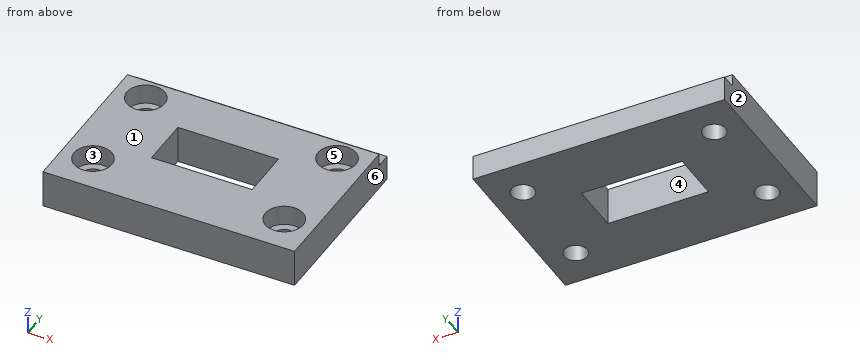
from build123d import *

# Parameters (mm, degrees)
SKETCH_1_W          = 100
SKETCH_1_H          = 70
EXTRUDE_1_DEPTH     = 15
SKETCH_2_W          = 100
SKETCH_2_H          = 6
CUT_EXTRUDE_1_DEPTH = 5
SKETCH_3_W          = 40
SKETCH_3_H          = 20
CUT_EXTRUDE_2_DEPTH = 63.84902545
SKETCH_4_R          = 7.5
CUT_EXTRUDE_3_DEPTH = 8
SKETCH_5_R          = 4.5
CUT_EXTRUDE_4_DEPTH = 63.84902545


with BuildPart() as part:
    # 草图1 → 凸台-拉伸1 (new body)
    with BuildSketch(Plane.XY):
        Rectangle(SKETCH_1_W, SKETCH_1_H)
    extrude(amount=EXTRUDE_1_DEPTH)

    # 草图2 → 切除-拉伸1 (cut)
    with BuildSketch(Plane.XY.offset(15)):
        with Locations((0, 32)):
            Rectangle(SKETCH_2_W, SKETCH_2_H)
    extrude(amount=-CUT_EXTRUDE_1_DEPTH, mode=Mode.SUBTRACT)

    # 草图3 → 切除-拉伸2 (cut, through all)
    with BuildSketch(Plane.XY):
        Rectangle(SKETCH_3_W, SKETCH_3_H)
    extrude(amount=CUT_EXTRUDE_2_DEPTH, mode=Mode.SUBTRACT)

    # 草图4 → 切除-拉伸3 (cut)
    with BuildSketch(Plane.XY.offset(15)):
        with Locations((38, 20)):
            Circle(SKETCH_4_R)
        with Locations((-38, 20)):
            Circle(SKETCH_4_R)
        with Locations((38, -20)):
            Circle(SKETCH_4_R)
        with Locations((-38, -20)):
            Circle(SKETCH_4_R)
    extrude(amount=-CUT_EXTRUDE_3_DEPTH, mode=Mode.SUBTRACT)

    # 草图5 → 切除-拉伸4 (cut, through all)
    with BuildSketch(Plane.XY.offset(15)):
        with Locations((38, 20)):
            Circle(SKETCH_5_R)
        with Locations((-38, 20)):
            Circle(SKETCH_5_R)
        with Locations((38, -20)):
            Circle(SKETCH_5_R)
        with Locations((-38, -20)):
            Circle(SKETCH_5_R)
    extrude(amount=-CUT_EXTRUDE_4_DEPTH, mode=Mode.SUBTRACT)


solid = part.part
The listing builds one solid part. Answer for the finished solid, in the listing's coordinates (mm). Face numbers are marked on the shaded views. A direction names the side the tool comes from. Coordinates: 2 decimals unless noted, no trailing zeros. Loops run counter-clockwise (first coordinate to the right, second up) from the corner with the lowest first, then second, coordinate; pieces in that order, holes last. Notation, with made-up numbers: (56, 44) -> (75, 44) arc R11 cw to (75, 53) -> close; hole circle Ø10 at (27.25, 20). An arc over 180 degrees is marked (long way). Answer in a Markdown table with one row per item. Add a question column.
1. For the marked faces 4, 5 and 6, determine the directions among +Z, -Z, +X, -X, +Y, -Y from which every point of the face is accessible in a straight line to the end or side of a thin tool.
2. The part is cut by section A-A, the plane x = -14. Write down the section's boundary in (y, z), then the cut area to 3 significant figures.
3. The part is cut by section B-B, the plane z = 8. Write down the section's boundary in (x, y).
4. Consider line 1 (Y direction, x = -38.5, z = 10.25); line 2 (Y direction, x = 38, z = 4); line 3 (Y direction, x = -13.5, z = 4). Determine where each line is inside the solid, lowest interval first. Write a range as [from, to].
5. The part is cut by section C-C, the plane y = -3. Write down the section's boundary in (x, z).
6. The part is cut by section D-D, the plane y = -18. Write down the section's boundary in (x, z).
7. Determine the mould class of the marked faces 1, 2 and 3 for opening direction X: +X half, -X half, draft (parallel to the pull), parting line (faces both ways), or undercut.
8. Flat-ended cylindrical pins translate along their axes: P1, Ø10.5, axis at x = -38, y = -20, coming from the +Z side; P2, Ø5, axis at x = -14.5, y = 33, coming from the +Z side; P3, Ø2.5, axis at x = 8.5, z = 13, coming from the +Y side. Find the tip coordinate at first contact, or state that the pin passes through.
Answer below:
| question | item | result |
|---|---|---|
| 1 | face 4 | +Z, -Z |
| 1 | face 5 | +Z |
| 1 | face 6 | +Z, -Z, +X, +Y, -Y |
| 2 | outline | (-35, 0) -> (-10, 0) -> (-10, 15) -> (-35, 15) -> close; (10, 0) -> (35, 0) -> (35, 10) -> (29, 10) -> (29, 15) -> (10, 15) -> close |
| 2 | area | 720 mm2 |
| 3 | outline | (-50, -35) -> (50, -35) -> (50, 35) -> (-50, 35) -> close; hole circle Ø15 at (-38, -20); hole circle Ø15 at (-38, 20); hole (-20, -10) -> (20, -10) -> (20, 10) -> (-20, 10) -> close; hole circle Ø15 at (38, -20); hole circle Ø15 at (38, 20) |
| 4 | line 1 | [-35, -27.48], [-12.52, 12.52], [27.48, 29] |
| 4 | line 2 | [-35, -24.5], [-15.5, 15.5], [24.5, 35] |
| 4 | line 3 | [-35, -10], [10, 35] |
| 5 | outline | (-50, 0) -> (-20, 0) -> (-20, 15) -> (-50, 15) -> close; (20, 0) -> (50, 0) -> (50, 15) -> (20, 15) -> close |
| 6 | outline | (-50, 0) -> (-42.03, 0) -> (-42.03, 7) -> (-45.23, 7) -> (-45.23, 15) -> (-50, 15) -> close; (-33.97, 0) -> (33.97, 0) -> (33.97, 7) -> (30.77, 7) -> (30.77, 15) -> (-30.77, 15) -> (-30.77, 7) -> (-33.97, 7) -> close; (42.03, 0) -> (50, 0) -> (50, 15) -> (45.23, 15) -> (45.23, 7) -> (42.03, 7) -> close |
| 7 | face 1 | draft |
| 7 | face 2 | -X half |
| 7 | face 3 | undercut |
| 8 | P1 | z = 7 |
| 8 | P2 | z = 10 |
| 8 | P3 | y = 29 |
